Build history of the part. All positions in model axes, mm. Face numbers are marked on the shaded views. A direction names the side the tool comes from. Round coordinates to 2 decimals unless told otherwise and drop trailing zeros. Loops run counter-clockwise (first coordinate to the right, second up) from the corner with the lowest first, then second, coordinate; pieces in that order, holes last. Notation, with made-up numbers: M -2,73.25 L 29,73.25 A22 ccw 29,90.25 Z; hole C 80.5,81 d8. An arc over 180 degrees is marked long. One line per item, written item: value.
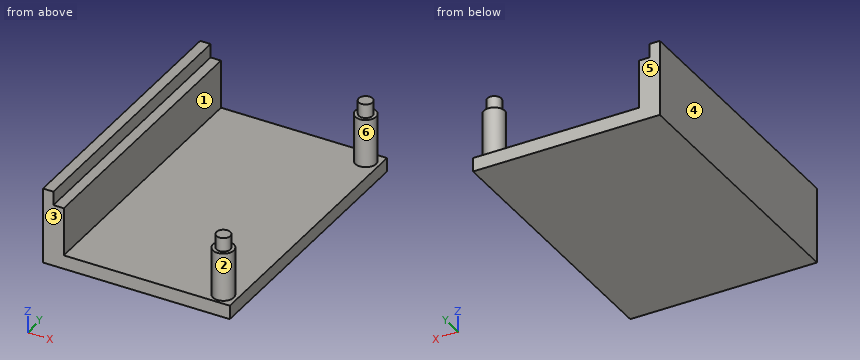
```python
from build123d import *

# Parameters (mm, degrees)
F0_W     = 24
F0_H     = 40
F0_R     = 1.5
F0_W_2   = 3
F1_DEPTH = 2
F2_DEPTH = 9
F3_DEPTH = 9
F4_W     = 1.5
F4_H     = 40
F4_R     = 1
F5_DEPTH = 2


with BuildPart() as f1:
    # F0 (on Top) → F1 (new body)
    with BuildSketch(Plane.XY):
        with Locations((-24.2441255752, 2.3181930908)):
            Rectangle(F0_W, F0_H)
        with Locations((-14.2441255752, -15.7818069092)):
            Circle(F0_R, mode=Mode.SUBTRACT)
        with Locations((-14.2441255752, 20.4181930908)):
            Circle(F0_R, mode=Mode.SUBTRACT)
        with Locations((-37.7441255752, 2.3181930908)):
            Rectangle(F0_W_2, F0_H)
        with Locations((-14.2441255752, 20.4181930908)):
            Circle(F0_R)
        with Locations((-14.2441255752, -15.7818069092)):
            Circle(F0_R)
    extrude(amount=F1_DEPTH)

    # F0 (on Top) → F2 (join)
    with BuildSketch(Plane.XY):
        with Locations((-37.7441255752, 2.3181930908)):
            Rectangle(F0_W_2, F0_H)
    extrude(amount=F2_DEPTH)

    # F0 (on Top) → F3 (join, through all)
    with BuildSketch(Plane.XY):
        with Locations((-14.2441255752, 20.4181930908)):
            Circle(F0_R)
        with Locations((-14.2441255752, -15.7818069092)):
            Circle(F0_R)
    extrude(amount=F3_DEPTH)

    # F4 (on face) → F5 (join)
    with BuildSketch(Plane.XY.offset(9)):
        with Locations((-38.4941255752, 2.3181930908)):
            Rectangle(F4_W, F4_H)
        with Locations((-14.2441255752, 20.4181930908)):
            Circle(F4_R)
        with Locations((-14.2441255752, -15.7818069092)):
            Circle(F4_R)
    extrude(amount=F5_DEPTH)


solid = f1.part
```
Item 1: Slice it at D-D, the plane z = 9.75. Give the cut face in (x, y).
Check values:
outline: M -39.24,-17.68 L -37.74,-17.68 L -37.74,22.32 L -39.24,22.32 Z; C -14.24,-15.78 d2; C -14.24,20.42 d2
Item 2: Pull direction X, two halves, no side cores. Call the marked faces 4, 5 and 6: pulls with the +X half, pulls with the -X half, needs draft (parallel to the pull), parting line crosses it, or undercut.
Check values:
face 4: pulls with the -X half
face 5: needs draft
face 6: undercut
Item 3: Slice it at B-B, the plane z = 5.5. Give the cut face in (x, y), and give its area (3 significant figures).
Check values:
outline: M -39.24,-17.68 L -36.24,-17.68 L -36.24,22.32 L -39.24,22.32 Z; C -14.24,-15.78 d3; C -14.24,20.42 d3
area: 134 mm2
Item 4: Slice it at C-C, the plane x = -16.75. Give the cut face in (y, z), and give its area (3 significant figures).
Check values:
outline: M -17.68,0 L 22.32,0 L 22.32,2 L -17.68,2 Z
area: 80.0 mm2
Item 5: Wall check: line 1 along Z through (x, y) = (-18.75, -7); line 2 along X through (y, z) = (-6, 7.75); line 3 along X through (y, z) = (-13, 9.5). Give the ranges that are in metal, low to high.
Check values:
line 1: z = 0 to 2
line 2: x = -39.24 to -36.24
line 3: x = -39.24 to -37.74
Item 6: Slice it at A-A, the plane y = 10.5. Give the cut face in (x, z), and give its area (3 significant figures).
Check values:
outline: M -39.24,0 L -12.24,0 L -12.24,2 L -36.24,2 L -36.24,9 L -37.74,9 L -37.74,11 L -39.24,11 Z
area: 78.0 mm2
Item 7: Which spindle directions (+Z, -Z, +X, -X, +Y, -Y) get a long thin tool onto all of the face, cutting with end or side? Do the marked faces 1, 2 and 3. Say none if no direction does.
Check values:
face 1: +Z, +Y, -Y
face 2: +Z
face 3: +Z, -Z, +X, -X, -Y
Item 8: Drop flat-ended pins along their axis: P1, Ø3, axis at x = -32, y = -3.5, coming from the +Z side; P2, Ø2, axis at y = -3.5, z = 5.5, coming from the +X side; P3, Ø1.5, axis at x = -16, z = 4.5, coming from the +Y side. Give the stop position or say it passes through.
Check values:
P1: stops at z = 2
P2: stops at x = -36.24
P3: stops at y = 21.53
